Check sheet for the modelled part. Datum: model origin and axes. Units: mm. A direction names the side the tool comes from. Give positions to 0.01 mm unless a question says otherwise; leave off trailing zeros. Loops run counter-clockwise (first coordinate to the right, second up) from the corner with the lowest first, then second, coordinate; pieces in that order, holes last. Notation, with made-up numbers: M -1,-26.75 L 29,-26.75 A19 cw 29,-20.75 Z; hole C 48,-0.5 d1. An arc over 180 degrees is marked long. Put each result on its own line as item: value. Start each with the question number.
```python
from build123d import *

# Parameters (mm, degrees)
SKETCH_2_R          = 3
CUT_EXTRUDE_1_DEPTH = 30.891470355
CHAMFER_1_SIZE      = 0.25
HOLE_WIZARD_M3_1_D  = 2.5


# Read off the part's stored shape, not the designer's step: M5 螺纹孔1
with BuildPart() as part:
    # 草图1 → 旋转1 (revolve)
    with BuildSketch(Plane(origin=(0, 0, 0), x_dir=(0, 0, -1), z_dir=(1, 0, 0)), mode=Mode.PRIVATE) as revolve_1_sk:
        Polygon((0, 0), (0, 8), (5.1, 8), (5.1, 13.5), (9.7, 13.5), (9.7, 8), (23, 8), (23, 0), align=None)
    revolve(revolve_1_sk.sketch.rotate(Axis((0, 0, 81.160359106), (0, 0, -1)), 90), axis=Axis((0, 0, 81.160359106), (0, 0, -1)))

    # 草图2 → 切除-拉伸1 (cut, through all)
    with BuildSketch(Plane(origin=(0, 0, -23), x_dir=(-1, 0, 0), z_dir=(0, 0, -1))):
        Circle(SKETCH_2_R)
    extrude(amount=-CUT_EXTRUDE_1_DEPTH, mode=Mode.SUBTRACT)

    # M5 螺纹孔1 outline → M5 螺纹孔1 (revolve, cut)
    with BuildSketch(Plane.XY.offset(-19)):
        Polygon((2.52511429, 8.00011429), (0, 8.00011429), (0, 2.141949197), (2.1, 2.141949197), (2.1, 7.575), align=None)
    revolve(axis=Axis((0, 0, -19), (0, 1, 0)), mode=Mode.SUBTRACT)

    # Hole Wizard M5 _1 2 outline → Hole Wizard M5 _1 2 (revolve, cut)
    with BuildSketch(Plane(origin=(0, 0, -19), x_dir=(0.49999999999999767, 0.86602540378444, 0), z_dir=(0, 0, -1))):
        Polygon((2.525122236, 8.000122236), (0, 8.000122236), (0, 2.1419531), (2.1, 2.1419531), (2.1, 7.575), align=None)
    revolve(axis=Axis((0, 0, -19), (0.8660254037844403, -0.4999999999999978, 0)), mode=Mode.SUBTRACT)

    # 倒角1
    chamfer_1_edges = [part.edges().sort_by_distance(p)[0] for p in [
        (3, 0, -23),
        (-8, 0, -23),
        (-8, 0, 0),
    ]]
    chamfer(chamfer_1_edges, length=CHAMFER_1_SIZE)

    # M3 螺纹孔1 (through all)
    with Locations(Plane(origin=(-11.5, 0, -5.1), x_dir=(1, 0, 0), z_dir=(0, 0, 1))):
        with Locations((0, 0), (17.25, -9.959292144), (17.25, 9.959292144), (1.540707856, 5.75), (11.5, -11.5), (21.459292144, 5.75)):
            Hole(HOLE_WIZARD_M3_1_D / 2)


solid = part.part
```
Q1. Section check A-A, the plane x = 0. Give the number of separate pieces and of enclosed holes in the cut face, then the cut area to 3 significant figures.
Q2. Mould release check, pull along Z, two halves, no side actions. Record for faces 1 (the face through (2.003, 4.897, -19.631)), 2 (the face through (6, 6, -9.7)), 3 (the face through (7, -10, -7)): pulls with the +Z half, pulls with the -Z half, needs draft (parallel to the pull), parting line crosses it, or undercut.
Q3. Section check B-B, the plane y = -9.5. Record the cut outline in (x, z), then the cut area to 3 significant figures.
Q4. Access from +Z, -Z, +X, -X, +Y, -Y to the whole of each face (thin tool, end or side, straight path). Record for faces 4 (the face through (-5.9, -5.4, -16.3)), 5 (the face through (-6, 6, -5.1)), 6 (the face through (5.24, -0.71, -18.37)).
Q5. Section check D-D, the plane z = -11.75. Record the cut outline in (x, y).
Q6. Depth check by flat-ended pin: P1, Ø12, axis at y = 9, z = -6.5, coming from the -X side; P2, Ø3, axis at x = 9.96, y = 5.75, coming from the -Z side; P3, Ø8, axis at x = 4.5, z = -11.5, coming from the +Y side. Enter the tip coordinate at first touch or a pass-through.
Q7. Thickness scan on line 1 along Z through (x, y) = (-11.75, 3.5); line 2 along Y through (x, z) = (5.75, -6.45); line 3 along Z through (x, y) = (0.5, 4.5). Record the ranges inside material, lowest first. Write a range as [from, to].
Found:
1. separate pieces: 4
1. enclosed holes: 0
1. area: 248 mm^2
2. face 1: undercut
2. face 2: pulls with the -Z half
2. face 3: needs draft
3. outline: M -9.59,-9.7 L 4.59,-9.7 L 4.59,-5.1 L -9.59,-5.1 Z; M 6.91,-9.7 L 9.59,-9.7 L 9.59,-5.1 L 6.91,-5.1 Z
3. area: 77.5 mm^2
4. face 4: -Z
4. face 5: +Z
4. face 6: none
5. outline: C 0,0 d16; hole C 0,0 d6
6. P1: stops at x = -13.16
6. P2: stops at z = -9.7
6. P3: stops at y = 13.47
7. line 1: z = [-9.7, -5.1]
7. line 2: y = [-12.21, -11.21], [-8.71, 8.71], [11.21, 12.21]
7. line 3: z = [-23, -21.04], [-16.96, 0]
